The model under review builds one solid part; all positions refer to its coordinate system, in mm. Face numbers are marked on the shaded views. A direction names the side the tool comes from. Round coordinates to 2 decimals unless told otherwise and drop trailing zeros. Write each loop counter-clockwise with the first axis right and the second up, starting at its lowest first coordinate (ties: lowest second). Pieces come first, ordered by that corner, then holes. Notation, with made-up numbers: (50.5, 37) -> (63.5, 37) arc R18 cw to (63.5, 62) -> close; hole circle Ø1 at (78, 67.25). An arc over 180 degrees is marked (long way). Return JSON: item names as keys, results as strings. Group by question number.
1. Take a section at C-C, the plane z = 4.5. Write out the cut boundary in (x, y), then the cut area to 3 significant figures.
2. Mouldability with a two-part tool opening along Y and no side actions: class the marked faces 1, 2 and 3 as pulls with the +Y half, pulls with the -Y half, needs draft (parallel to the pull), parting line crosses it, or undercut.
3. Clearance check with flat-ended pins moving along their axes: P1, Ø4, axis at y = -5, z = 4.5, coming from the -X side; P2, Ø2.5, axis at x = 2, y = 1, coming from the +Z side; P3, Ø2.5, axis at x = 0, y = 0, coming from the +Z side; P4, Ø3, axis at x = 3.5, z = 4, coming from the -Y side. State where each tip first meets the part, or that it passes through.
4. Take a section at D-D, the plane z = 0.5. Write out the cut boundary in (x, y).
5. Take a section at A-A, the plane x = 0. Write out the cut boundary in (y, z), then the cut area to 3 significant figures.
6. For line 1 along Y through (x, z) = (0, 3.5); line 2 along Y through (x, z) = (0, 2.35); line 3 along X through (y, z) = (1, 0.5), list the stretches that pass through material, from the lowest coordinate up. Write a range as from..to.
7. Tool access review of the marked faces 4 and 5: name each direction out of +Z, -Z, +X, -X, +Y, -Y from which nothing blocks a thin tool from reaching the whole face with its end or side.
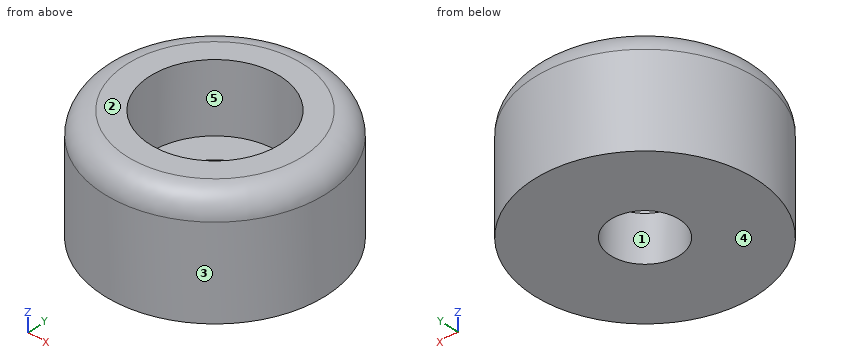
from build123d import *

# Parameters (mm, degrees)
F4_R     = 7.25
F4_R_2   = 4.25
F5_DEPTH = 7.5
F4_R_3   = 2.25
F6_DEPTH = 3
F7_R     = 1.5


# Not quite as in the source:
# - a feature of the source that left no trace in its solid (it failed there, or was rolled back) is left out


with BuildPart() as f5:
    # F4 (on Top) → F5 (new body)
    with BuildSketch(Plane.XY):
        Circle(F4_R)
        Circle(F4_R_2, mode=Mode.SUBTRACT)
    extrude(amount=F5_DEPTH)

    # F4 (on Top) → F6 (join)
    with BuildSketch(Plane.XY):
        Circle(F4_R_2)
        Circle(F4_R_3, mode=Mode.SUBTRACT)
    extrude(amount=F6_DEPTH)

    # F7
    f7_edges = [f5.edges().sort_by_distance(p)[0] for p in [
        (-7.25, 0, 7.5),
    ]]
    fillet(f7_edges, radius=F7_R)


solid = f5.part
Output:
{
 "1": {"outline": "circle Ø14.5 at (0, 0); hole circle Ø8.5 at (0, 0)", "area": "108 mm^2"},
 "2": {"face 1": "undercut", "face 2": "needs draft", "face 3": "parting line crosses it"},
 "3": {"P1": "stops at x = -6.6", "P2": "stops at z = 3", "P3": "passes through", "P4": "stops at y = -6.97"},
 "4": {"outline": "circle Ø14.5 at (0, 0); hole circle Ø4.5 at (0, 0)"},
 "5": {"outline": "(-7.25, 0) -> (-2.25, 0) -> (-2.25, 3) -> (-4.25, 3) -> (-4.25, 7.5) -> (-5.75, 7.5) arc R1.5 ccw to (-7.25, 6) -> close; (2.25, 0) -> (7.25, 0) -> (7.25, 6) arc R1.5 ccw to (5.75, 7.5) -> (4.25, 7.5) -> (4.25, 3) -> (2.25, 3) -> close", "area": "56.0 mm^2"},
 "6": {"line 1": "y = -7.25..-4.25, 4.25..7.25", "line 2": "y = -7.25..-2.25, 2.25..7.25", "line 3": "x = -7.18..-2.02, 2.02..7.18"},
 "7": {"face 4": "-Z, +X, -X, +Y, -Y", "face 5": "+Z"}
}
